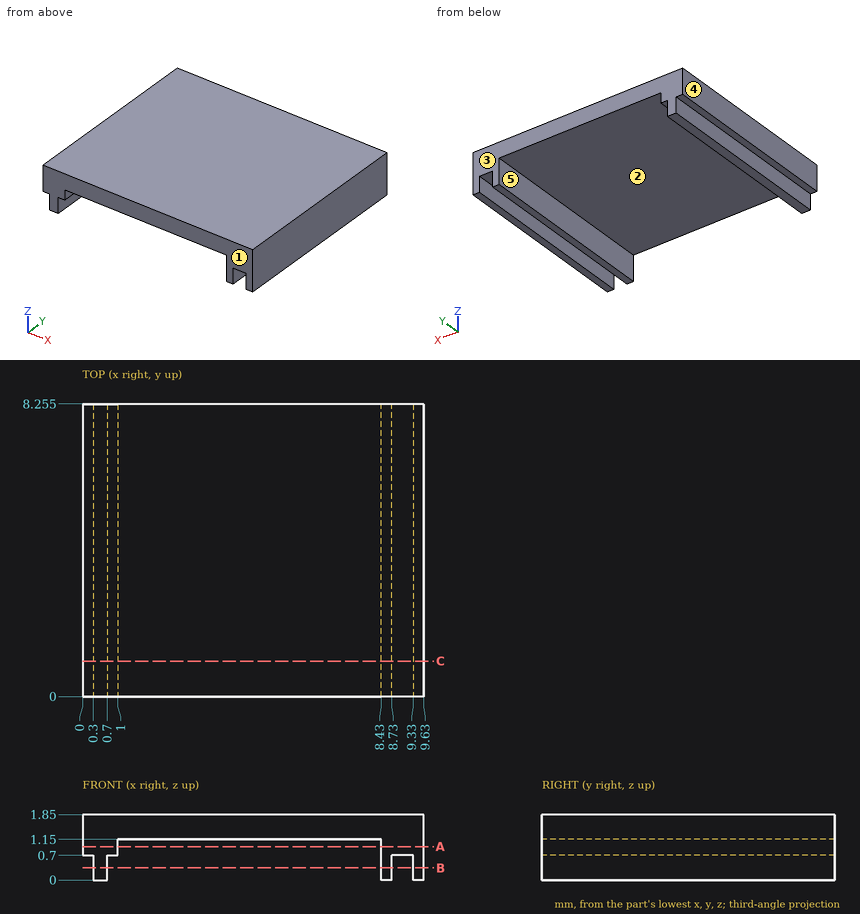
The figure shows three views and two pictorial views of one solid part (mm, origin at its lowest corner). Answer the questions. A direction names the side the tool comes from. Coordinates: 2 decimals unless noted, no trailing zeros. Loops run counter-clockwise (first coordinate to the right, second up) from the corner with the lowest first, then second, coordinate; pieces in that order, holes last. Notation, with made-up numbers: M 54,38.5 L 112,38.5 A29 cw 112,65.5 Z; hole C 35,35.25 d9. An arc over 180 degrees is marked long. Answer as CSV lines item,"result". Start each with the question number.
(1) The part is cut by section C-C (y = 1). Give the vertices of the cut face in (x, z).
(2) Find the intervals of material crossed by L1, parallel to X at y = 0.5, z = 0.65; L2, parallel to X at y = 0.5, z = 0.85; L3, parallel to Z at x = 6.75, y = 1.75, in increasing order. Write a range as [from, to].
(3) The mould has two halves that part along X. Classify the marked faces 3, 4 and 5: pulls with the +X half, pulls with the -X half, needs draft (parallel to the pull), parting line crosses it, or undercut.
(4) Given pin 1 (0.6 mm diameter, centred on y = 4.5, z = 0, fed in from -X); pin 2 (4 mm diameter, centred on x = 3.5, y = 5, fed in from -Z), each flat-ended and moving along its own axis, determine where each tip first touches the part or whether it passes through.
(5) The part is cut by section B-B (z = 0.35). State how many separate pieces and enclosed holes the cut face has.
(6) For the marked faces 1 and 2, determine the directions among +Z, -Z, +X, -X, +Y, -Y from which every point of the face is accessible in a straight line to the end or side of a thin tool.
(7) The part is cut by section A-A (z = 0.95). Give the vertices of the cut face in (x, y) (1 decimal).
Determined:
1,outline,"M 0,0.7 L 0.3,0.7 L 0.3,0 L 0.7,0 L 0.7,0.7 L 1,0.7 L 1,1.15 L 8.43,1.15 L 8.43,0 L 8.73,0 L 8.73,0.7 L 9.33,0.7 L 9.33,0 L 9.63,0 L 9.63,1.85 L 0,1.85 Z"
2,L1,"[0.3, 0.7], [8.43, 8.73], [9.33, 9.63]"
2,L2,"[0, 1], [8.43, 9.63]"
2,L3,"[1.15, 1.85]"
3,face 3,"needs draft"
3,face 4,"pulls with the -X half"
3,face 5,"undercut"
4,pin 1,"x = 0.3"
4,pin 2,"z = 1.15"
5,separate pieces,"3"
5,enclosed holes,"0"
6,face 1,"+Z, -Z, +X, -X, -Y"
6,face 2,"-Z, +Y, -Y"
7,outline,"M 0,0 L 1,0 L 1,8.3 L 0,8.3 Z; M 8.4,0 L 9.6,0 L 9.6,8.3 L 8.4,8.3 Z"
